Source: CAD feature listing. Evaluate the final solid. Frame: model axes, mm. A direction names the side the tool comes from. Coordinates: 2 decimals unless noted, no trailing zeros. Loops run counter-clockwise (first coordinate to the right, second up) from the corner with the lowest first, then second, coordinate; pieces in that order, holes last. Notation, with made-up numbers: (84, -23) -> (125, -23) arc R17 cw to (125, 7) -> close; hole circle Ø2 at (11.5, -5.5). An arc over 180 degrees is marked (long way). One line per question, with ' | ' between items. Start each with the question number.
```python
from build123d import *

# Parameters (mm, degrees)
BOSS_EXTRUDE2_DEPTH = 5
BOSS_EXTRUDE3_DEPTH = 2
SKETCH4_R           = 1
CUT_EXTRUDE1_DEPTH  = 96.580030811
FILLET1_R           = 1
FILLET2_R           = 1
SKETCH5_R           = 2.5
CUT_EXTRUDE2_DEPTH  = 97.594732206
BOSS_EXTRUDE4_DEPTH = 5


with BuildPart() as part:
    # Sketch1 → Boss-Extrude2 (new, symmetric)
    with BuildSketch(Plane(origin=(0, 0, 0), x_dir=(1, 0, 0), z_dir=(0, 1, 0))):
        with BuildLine():
            Line((-49, 0), (49, 0))
            Line((49, 0), (55, 0))
            Line((55, 0), (55, 10))
            Line((55, 10), (49, 10))
            Line((49, 10), (-48.597064799, 10))
            ThreePointArc((-48.597064799, 10), (-51.770174838, 10.516784686), (-54.615321941, 12.013725463))
            Line((-54.615321941, 12.013725463), (-78.198331144, 29.785292532))
            ThreePointArc((-78.198331144, 29.785292532), (-79.051875275, 30.234374765), (-80.003808287, 30.389410171))
            Line((-80.003808287, 30.389410171), (-88.011381516, 30.389410171))
            ThreePointArc((-88.011381516, 30.389410171), (-88.959703047, 29.706721175), (-88.61320723, 28.590782717))
            Line((-88.61320723, 28.590782717), (-52.009128571, 1.006862732))
            ThreePointArc((-52.009128571, 1.006862732), (-50.586555019, 0.258392343), (-49, 0))
        make_face()
    extrude(amount=BOSS_EXTRUDE2_DEPTH, both=True)

    # Sketch3 → Boss-Extrude3 (add)
    with BuildSketch(Plane.XY):
        Polygon((55, -5), (41, -5), (41, -10), (43, -10), (43, -17), (53, -17), (53, -10), (55, -10), align=None)
    boss_extrude3 = extrude(amount=-BOSS_EXTRUDE3_DEPTH)

    # Sketch4 → Cut-Extrude1 (cut, through all)
    with BuildSketch(Plane.XY):
        with BuildLine():
            Line((55, -10), (55, -9))
            ThreePointArc((55, -9), (54.707106781, -9.707106781), (54, -10))
            Line((54, -10), (55, -10))
        make_face()
        with BuildLine():
            Line((53, -14.5), (53, -10))
            Line((53, -10), (49.535533906, -10))
            Line((49.535533906, -10), (52.267766953, -12.732233047))
            ThreePointArc((52.267766953, -12.732233047), (52.809698831, -13.543291419), (53, -14.5))
        make_face()
        with BuildLine():
            Line((53, -17), (53, -14.5))
            ThreePointArc((53, -14.5), (52.267766953, -16.267766953), (50.5, -17))
            Line((50.5, -17), (53, -17))
        make_face()
        with BuildLine():
            ThreePointArc((42, -10), (41.292893219, -9.707106781), (41, -9))
            Line((41, -9), (41, -10))
            Line((41, -10), (42, -10))
        make_face()
        with BuildLine():
            Line((43, -17), (50.5, -17))
            ThreePointArc((50.5, -17), (49.441268366, -16.764748844), (48.581791004, -16.103269862))
            Line((48.581791004, -16.103269862), (43, -10))
            Line((43, -10), (43, -17))
        make_face()
        with Locations((50.5, -14.5)):
            Circle(SKETCH4_R)
    cut_extrude1 = extrude(amount=-CUT_EXTRUDE1_DEPTH, mode=Mode.SUBTRACT)

    # Mirror1: Boss-Extrude3, Cut-Extrude1 across plane
    add(boss_extrude3.mirror(Plane.XY.offset(-5)))
    add(cut_extrude1.mirror(Plane.XY.offset(-5)), mode=Mode.SUBTRACT)

    # Fillet1
    fillet1_edges = [part.edges().sort_by_distance(p)[0] for p in [
        (-4, -5, 0),
        (-50.586555019, -5, -0.258392343),
        (-70.3111679, -5, -14.798822724),
        (-88.959703047, -5, -29.706721175),
        (-84.007594901, -5, -30.389410171),
        (-79.051875275, -5, -30.234374765),
        (-66.406826543, -5, -20.899508998),
        (-3.7985324, -5, -10),
        (-51.770174838, -5, -10.516784686),
    ]]
    fillet(fillet1_edges, radius=FILLET1_R)

    # Fillet2
    fillet2_edges = [part.edges().sort_by_distance(p)[0] for p in [
        (3.2014676, 5, -10),
        (-51.770174838, 5, -10.516784686),
        (-66.406826543, 5, -20.899508998),
        (-79.051875275, 5, -30.234374765),
        (-84.007594901, 5, -30.389410171),
        (-88.959703047, 5, -29.706721175),
        (-70.3111679, 5, -14.798822724),
        (-50.586555019, 5, -0.258392343),
        (3, 5, 0),
    ]]
    fillet(fillet2_edges, radius=FILLET2_R)

    # Sketch5 → Cut-Extrude2 (cut, through all)
    with BuildSketch(Plane(origin=(0, 5, 0), x_dir=(1, 0, 0), z_dir=(0, 1, 0))):
        with Locations(Location((30, 5, 0), (0, 0, 270))):
            Circle(SKETCH5_R)
        with Locations(Location((-35, 5, 0), (0, 0, 270))):
            Circle(SKETCH5_R)
    extrude(amount=-CUT_EXTRUDE2_DEPTH, mode=Mode.SUBTRACT)

    # Sketch6 → Boss-Extrude4 (add, symmetric)
    with BuildSketch(Plane(origin=(0, 0, 0), x_dir=(0, 0, -1), z_dir=(1, 0, 0))):
        with BuildLine():
            Line((0, 2.75), (0, -2.75))
            Line((0, -2.75), (-2.75, -2.75))
            Line((-2.75, -2.75), (-2.75, -2.25))
            ThreePointArc((-2.75, -2.25), (-0.5, 0), (-2.75, 2.25))
            ThreePointArc((-2.75, 2.25), (-4.340990258, 1.590990258), (-5, 0))
            Line((-5, 0), (-5.5, 0))
            ThreePointArc((-5.5, 0), (-4.694543648, 1.944543648), (-2.75, 2.75))
            Line((-2.75, 2.75), (0, 2.75))
        make_face()
    extrude(amount=BOSS_EXTRUDE4_DEPTH, both=True)


solid = part.part
```
(1) Contact query for flat-ended pins moving along their axis: pin 1 Ø3 at (x, y) = (50.5, -14.5) entering from +Z; pin 2 Ø1 at (x, y) = (-54.5, -1) entering from -Z; pin 3 Ø1.6 at (y, z) = (-0.5, 2) entering from -X; pin 4 Ø5 at (y, z) = (0, 2.75) entering from +X. Output: stop coordinate, or through.
(2) Draft query along Z for faces 4 (the cylindrical face through (32.11, 0.07, -3.66)), 5 (the flat face through (5, 0.828, 0.496)), 6 (the cylindrical face through (0.07, 1.92, 4.72)). Return one class per face: pulls with the +Z half, pulls with the -Z half, needs draft (parallel to the pull), parting line crosses it, or undercut.
(3) Cut plane D-D, the plane z = -5. State how many separate pieces and enclosed holes the cut face has, and give its area (3 significant figures).
(4) Ray query, L1, parallel to Y at x = 50.5, z = -0.7; L2, parallel to X at y = -2.5, z = -5; L3, parallel to Y at x = 17, z = -3. Return the intervals inside material, ascending.
(5) Cut plane B-B, the plane x = -35. Return the cut outline in (y, z), and give its area (3 significant figures).
(6) Cut plane C-C, the plane x = -11.5. Return the cut outline in (y, z), and give its area (3 significant figures).
(7) Access query for faces 1 (the flat face through (-5, 0.828, 0.496)), 2 (the flat face through (0, -2.75, 1)), 3 (the flat face through (-84, 0, -30.389)). Directions: +Z, -Z, +X, -X, +Y, -Y. A direction counts if a zero-diameter tool reaches every point of the face in a straight line with its end or side. Return the directions, or none.
(8) Cut plane A-A, the plane y = -7. Return the cut outline in (x, z).
Here are the results:
1) pin 1: stops at z = 0 | pin 2: stops at z = -12.3 | pin 3: passes through | pin 4: stops at x = 5
2) face 4: undercut | face 5: needs draft | face 6: pulls with the +Z half
3) separate pieces: 3 | enclosed holes: 0 | area: 1,020 mm2
4) L1: y = -17 to -15.5, -13.5 to -10.96, -10 to 4.95 | L2: x = -57.31 to -37.5, -32.5 to 27.5, 32.5 to 55 | L3: y = -5 to 5
5) outline: (-5, -9) arc R1 ccw to (-4, -10) -> (4, -10) arc R1 ccw to (5, -9) -> (5, -7.5) -> (-5, -7.5) -> close; (-5, -2.5) -> (5, -2.5) -> (5, -1) arc R1 ccw to (4, 0) -> (-4, 0) arc R1 ccw to (-5, -1) -> close | area: 49.1 mm2
6) outline: (-5, -9) arc R1 ccw to (-4, -10) -> (4, -10) arc R1 ccw to (5, -9) -> (5, -1) arc R1 ccw to (4, 0) -> (-4, 0) arc R1 ccw to (-5, -1) -> close | area: 99.1 mm2
7) face 1: +Z, -X, +Y, -Y | face 2: +Z, +X, -X, -Y | face 3: -Z, +X, -X, +Y, -Y
8) outline: (41, -10) -> (55, -10) -> (55, -8) -> (41, -8) -> close; (41, -2) -> (55, -2) -> (55, 0) -> (41, 0) -> close
